Can you work these out from the model? Positions are in its coordinate system, mm. A direction names the side the tool comes from. Coordinates: 2 decimals unless noted, no trailing zeros. Order: outer loops, then holes, each group sorted by start corner. A loop starts at its lowest first (then second) coordinate and runs counter-clockwise, first axis right, second up. Notation, with made-up numbers: (9, 62) -> (54, 62) arc R13 ccw to (54, 70) -> close; hole circle Ø2 at (24, 79). An arc over 180 degrees is marked (long way). Answer in a Markdown table with one row per item.
```python
from build123d import *

# Parameters (mm, degrees)
F1_DEPTH = 25
F2_T     = -6
F4_R     = 15.0616711188
F5_DEPTH = 12.5


with BuildPart() as f1:
    # F0 (on Top) → F1 (new body)
    with BuildSketch(Plane.XY):
        Polygon((74.3237713212, 43.4907621871), (-0.5022192234, 86.1116551627), (-74.8259905445, 42.6208929757), (-74.3237713212, -43.4907621871), (0.5022192234, -86.1116551627), (74.8259905445, -42.6208929757), align=None)
        Polygon((0.4048665783, -69.4193482725), (-60.3213524073, 34.3590493943), (59.916485829, 35.0602988782), align=None, mode=Mode.SUBTRACT)
    extrude(amount=F1_DEPTH)

    # F2
    f2_openings = [f1.faces().sort_by_distance(p)[0] for p in [
        (35.781524, 62.818673, 25),
    ]]
    offset(amount=F2_T, openings=f2_openings, kind=Kind.INTERSECTION)

    # F4 (on face) → F5 (join, symmetric)
    with BuildSketch(Plane.XY.offset(6)):
        with Locations((-0.461813338, 58.4901720285)):
            Circle(F4_R)
        with Locations((50.8848815174, -28.8451439318)):
            Circle(F4_R)
        with Locations((-50.4230681795, -29.6450280968)):
            Circle(F4_R)
    extrude(amount=F5_DEPTH, both=True)


with BuildPart() as f1b:
    # F0 (on Top) → F1, piece 2 (new body)
    with BuildSketch(Plane.XY):
        Polygon((29.9582429145, 17.5301494391), (-30.1606762036, 17.1795246971), (0.2024332891, -34.7096741362), align=None)
    extrude(amount=F1_DEPTH)


solid = f1.part
```
(1) I need wall thicknesses on line 1 (X direction, y = -50, z = 21.5); line 2 (X direction, y = 62, z = 7.5); line 3 (Y direction, x = -52, z = 13). Which ranges of each line are inside material? Lowest first, please. Write a range as [from, to].
Response values:
| item | result |
|---|---|
| line 1 | [-62.9, -50.77], [-17.91, -10.96], [11.47, 18.37], [50.34, 62.22] |
| line 2 | [-41.71, -29.83], [-15.11, 14.19], [29.71, 41.83] |
| line 3 | [-56.21, -49.3], [-44.62, -14.67], [8.26, 20.14], [34.41, 40.41], [49.03, 55.98] |
(2) On a 3-axis mill with a long thin cutter (end or side, diameter ignored), from which of +Z, -Z, +X, -X, +Y, -Y can I reach the whole of each face in a straight line? I mean faces 1 (the flat face through (30.577, -16.448, 12.325)), 2 (the flat face through (-51, -29, -6.5)), 3 (the flat face through (-1, 59, 18.5)). Say none if no direction works.
Response values:
| item | result |
|---|---|
| face 1 | +Z, -Z |
| face 2 | -Z, +X, -X, +Y, -Y |
| face 3 | +Z |
(3) Suppose I cut it at C-C (y = -10). Please give me the cut outline in (x, z).
Response values:
| item | result |
|---|---|
| outline | (-74.52, 0) -> (-34.36, 0) -> (-34.36, 25) -> (-41.32, 25) -> (-41.32, 6) -> (-68.52, 6) -> (-68.52, 25) -> (-74.52, 25) -> close; (34.25, 0) -> (74.64, 0) -> (74.64, 25) -> (68.64, 25) -> (68.64, 6) -> (41.16, 6) -> (41.16, 25) -> (34.25, 25) -> close |
(4) Suppose I cut it at D-D (z = 20.5). Please give me the cut outline in (x, y), and give its area (3 significant figures).
Response values:
| item | result |
|---|---|
| outline | (-74.83, 42.62) -> (-74.32, -43.49) -> (0.5, -86.11) -> (74.83, -42.62) -> (74.32, 43.49) -> (-0.5, 86.11) -> close; hole (-68.79, 36.96) -> (-68.34, -39.99) -> (-1.48, -78.08) -> close; hole (-66.88, 40.32) -> (66.4, 41.1) -> (-0.46, 79.18) -> close; hole (-60.32, 34.36) -> (0.4, -69.42) -> (59.92, 35.06) -> close; hole (2.39, -78.05) -> (68.81, -39.19) -> (68.36, 37.76) -> close |
| area | 5,310 mm2 |
(5) Suppose I cut it at B-B (z = 10). Please give me the cut outline in (x, y), and give its area (3 significant figures).
Response values:
| item | result |
|---|---|
| outline | (-74.83, 42.62) -> (-74.32, -43.49) -> (0.5, -86.11) -> (74.83, -42.62) -> (74.32, 43.49) -> (-0.5, 86.11) -> close; circle Ø30.12 at (-50.42, -29.65); circle Ø30.12 at (-0.46, 58.49); circle Ø30.12 at (50.88, -28.85); hole (-68.79, 36.96) -> (-68.34, -39.99) -> (-1.48, -78.08) -> close; hole (-66.88, 40.32) -> (66.4, 41.1) -> (-0.46, 79.18) -> close; hole (-60.32, 34.36) -> (0.4, -69.42) -> (59.92, 35.06) -> close; hole (2.39, -78.05) -> (68.81, -39.19) -> (68.36, 37.76) -> close |
| area | 7,450 mm2 |
(6) Suppose I cut it at A-A (x = -9.5). Please give me the cut outline in (y, z), and give its area (3 significant figures).
Response values:
| item | result |
|---|---|
| outline | (-80.41, 0) -> (-52.49, 0) -> (-52.49, 25) -> (-64.37, 25) -> (-64.37, 6) -> (-73.51, 6) -> (-73.51, 25) -> (-80.41, 25) -> close; (34.66, 0) -> (46.44, 0) -> (46.44, -6.5) -> (70.54, -6.5) -> (70.54, 0) -> (80.85, 0) -> (80.85, 25) -> (73.89, 25) -> (73.89, 6) -> (70.54, 6) -> (70.54, 18.5) -> (46.44, 18.5) -> (46.44, 6) -> (40.66, 6) -> (40.66, 25) -> (34.66, 25) -> close |
| area | 1,510 mm2 |
(7) We'd pull the mould along Y, two halves only. Please class faces 4 (the flat face through (-34, -18, 0)), 5 (the flat face through (37.144, -64.671, 12.325)), 6 (the flat face through (-34.666, -21.366, 15.367)), 7 (the cylindrical face through (-3.727, 43.787, -3.204)): +Y half, -Y half, draft (parallel to the pull), parting line (faces both ways), or undercut.
Response values:
| item | result |
|---|---|
| face 4 | draft |
| face 5 | -Y half |
| face 6 | undercut |
| face 7 | parting line |
(8) Will these pins go through, and if not, where does the flat tip stop? pin 1 Ø9 at (x, y) = (-57.5, -30.5) entering from +Z; pin 2 Ø6 at (x, y) = (18, 31.5) entering from -Z; pin 3 Ø10 at (y, z) = (67, 10.5) entering from +X; pin 4 Ø12 at (x, z) = (-52, 5.5) entering from +Y.
Response values:
| item | result |
|---|---|
| pin 1 | z = 18.5 |
| pin 2 | through |
| pin 3 | x = 41.83 |
| pin 4 | y = 59.49 |
